from build123d import *

# Parameters (mm, degrees)
SKETCH004_R      = 2
PAD001_DEPTH     = 7
HOLE_D           = 5.5
HOLE_DEPTH       = 25
HOLE_CBORE_D     = 10
HOLE_CBORE_DEPTH = 3
FILLET_R         = 11


with BuildPart() as part:
    # Sketch004 → Pad001 (new body)
    with BuildSketch(Plane(origin=(0, 0, 0), x_dir=(-1, 0, 0), z_dir=(0, 0, -1))):
        Polygon((29, 10), (29, -30.5), (3, -30.5), (3, -10.3), (21, -10.3), (21, 10), align=None)
        with Locations((25, 6)):
            Circle(SKETCH004_R, mode=Mode.SUBTRACT)
        with Locations((25, -6)):
            Circle(SKETCH004_R, mode=Mode.SUBTRACT)
    extrude(amount=PAD001_DEPTH)

    # Hole
    with Locations(Plane.XY):
        with Locations((-15, -20.5)):
            CounterBoreHole(HOLE_D / 2, HOLE_CBORE_D / 2, HOLE_CBORE_DEPTH, depth=HOLE_DEPTH)

    # Fillet
    fillet_edges = [part.edges().sort_by_distance(p)[0] for p in [
        (-29, -30.5, -3.5),
        (-3, -30.5, -3.5),
    ]]
    fillet(fillet_edges, radius=FILLET_R)


with BuildPart() as part_1:
    # Body002 placement: moved
    add(part.part.moved(Location((-9.5, 0, -14))))


solid = part_1.part
Verification items for the finished model (mm, model axes). A direction names the side the tool comes from. Coordinates: 2 decimals unless noted, no trailing zeros. Write each loop counter-clockwise with the first axis right and the second up, starting at its lowest first coordinate (ties: lowest second). Pieces come first, ordered by that corner, then holes. Notation, with made-up numbers: (84, 74) - (139, 74) arc R27 cw to (139, 99) - close; hole circle Ø2 at (24, 29). An arc over 180 degrees is marked (long way). Answer as a JSON object with one key per item and string values.
(1) Mould release check, pull along Y, two halves, no side actions. Record for faces 4 (the flat face through (-26, -30.5, -17)), 5 (the flat face through (-22, -23, -17)), 6 (the flat face through (-12.5, -15, -17)): pulls with the +Y half, pulls with the -Y half, needs draft (parallel to the pull), parting line crosses it, or undercut.
Report:
{"face 4": "pulls with the -Y half", "face 5": "undercut", "face 6": "needs draft"}
(2) Cross-section at D-D on x = -34.5. Record the cut outline in (y, z).
Report:
{"outline": "(-27.99, -21) - (-8, -21) - (-8, -14) - (-27.99, -14) - close; (-4, -21) - (4, -21) - (4, -14) - (-4, -14) - close; (8, -21) - (10, -21) - (10, -14) - (8, -14) - close"}
(3) Cross-section at A-A on y = -6. Record the cut outline in (x, z).
Report:
{"outline": "(-38.5, -21) - (-36.5, -21) - (-36.5, -14) - (-38.5, -14) - close; (-32.5, -21) - (-30.5, -21) - (-30.5, -14) - (-32.5, -14) - close"}
(4) Cross-section at B-B on x = -24.5. Record the cut outline in (y, z).
Report:
{"outline": "(-30.5, -21) - (-23.25, -21) - (-23.25, -17) - (-25.5, -17) - (-25.5, -14) - (-30.5, -14) - close; (-17.75, -21) - (-10.3, -21) - (-10.3, -14) - (-15.5, -14) - (-15.5, -17) - (-17.75, -17) - close"}
(5) Cross-section at C-C on z = -15.5. Record the cut outline in (x, y), plus the area to 3 significant figures.
Report:
{"outline": "(-38.5, -19.5) arc R11 ccw to (-27.5, -30.5) - (-23.5, -30.5) arc R11 ccw to (-12.5, -19.5) - (-12.5, -10.3) - (-30.5, -10.3) - (-30.5, 10) - (-38.5, 10) - close; hole circle Ø4 at (-34.5, -6); hole circle Ø4 at (-34.5, 6); hole circle Ø10 at (-24.5, -20.5)", "area": "532 mm^2"}
(6) Tool access check on faces 1 (the flat face through (-34, 10, -17)), 2 (the flat face through (-30.5, 0, -17)), 3 (the cylindrical face through (-28.5, -23.5, -15.5)). Record the directions out of +Z, -Z, +X, -X, +Y, -Y that give a thin tool (end or side, any length) a straight path to the whole face; none if there is none.
Report:
{"face 1": "+Z, -Z, +X, -X, +Y", "face 2": "+Z, -Z, +X, +Y", "face 3": "+Z"}
(7) Thickness scan on line 1 along Y through (x, z) = (-24.5, -15.8); line 2 along Y through (x, z) = (-24.5, -18.55); line 3 along Y through (x, z) = (-34.5, -17.75). Record the ranges inside material, lowest first.
Report:
{"line 1": "-30.5 to -25.5, -15.5 to -10.3", "line 2": "-30.5 to -23.25, -17.75 to -10.3", "line 3": "-27.99 to -8, -4 to 4, 8 to 10"}
(8) Gauge pin test, flat ends, axial feed: pin 1 Ø1.5 at (x, z) = (-16, -15) entering from +Y; pin 2 Ø5 at (x, y) = (-24.5, -21) entering from +Z; pin 3 Ø3.5 at (x, y) = (-34.5, 6) entering from +Z. Record the tip position at first contact, or that the pin passes through.
Report:
{"pin 1": "y = -10.3", "pin 2": "z = -17", "pin 3": "through"}
